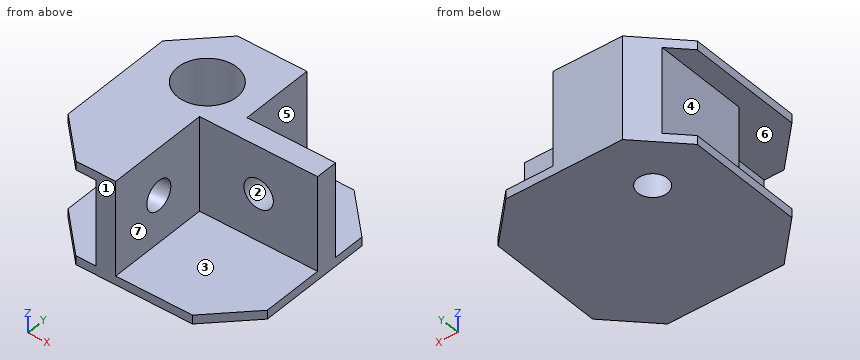
from build123d import *

# Parameters (mm, degrees)
F0_W      = 42.8625
F0_H      = 42.8625
F1_DEPTH  = 22.225
F2_SIZE   = 8.89
F3_W      = 25.4
F3_H      = 22.225
F4_DEPTH  = 20.32
F5_W      = 19.05
F5_H      = 15.875
F6_DEPTH  = 20.32
F8_D      = 12.7
F8_DEPTH  = 20.32
F8_TIP    = 3.8154649308
F9_W      = 14.1852621388
F9_H      = 18.415
F10_DEPTH = 17.78
F11_W     = 6.263975054
F11_H     = 18.415
F12_DEPTH = 25.0835
F14_D     = 6.35
F16_D     = 6.35


with BuildPart() as f1:
    # F0 (on Top) → F1 (new body)
    with BuildSketch(Plane.XY):
        Rectangle(F0_W, F0_H)
    extrude(amount=F1_DEPTH)

    # F2
    f2_edges = [f1.edges().sort_by_distance(p)[0] for p in [
        (-21.43125, -21.43125, 11.1125),
        (21.43125, -21.43125, 11.1125),
        (21.43125, 21.43125, 11.1125),
        (-21.43125, 21.43125, 11.1125),
    ]]
    chamfer(f2_edges, length=F2_SIZE)

    # F3 (on face) → F4 (cut)
    with BuildSketch(Plane.XY.offset(22.225)):
        with Locations((8.73125, -10.31875)):
            Rectangle(F3_W, F3_H)
    extrude(amount=-F4_DEPTH, mode=Mode.SUBTRACT)

    # F5 (on face) → F6 (cut)
    with BuildSketch(Plane.XY.offset(22.225)):
        with Locations((11.90625, 13.49375)):
            Rectangle(F5_W, F5_H)
    extrude(amount=-F6_DEPTH, mode=Mode.SUBTRACT)

    # F8
    with Locations(Plane.XY.offset(22.225)):
        with Locations((-8.73125, 8.73125)):
            Hole(F8_D / 2, depth=F8_DEPTH)
            with Locations((0, 0, -(F8_DEPTH + F8_TIP / 2))):  # 118° drill point
                Cone(0, F8_D / 2, F8_TIP, mode=Mode.SUBTRACT)

    # F9 (on face) → F10 (cut)
    with BuildSketch(Plane.XZ.offset(21.43125)):
        with Locations((-15.3476310694, 11.1125)):
            Rectangle(F9_W, F9_H)
    extrude(amount=-F10_DEPTH, mode=Mode.SUBTRACT)

    # F11 (on face) → F12 (cut, through all)
    with BuildSketch(Plane.XZ.offset(3.65125)):
        with Locations((-20.3739013523, 11.1125)):
            Rectangle(F11_W, F11_H)
    extrude(amount=-F12_DEPTH, mode=Mode.SUBTRACT)

    # F14 (through all)
    with Locations(Plane.YZ.offset(-3.96875)):
        with Locations((-10.00125, 12.065)):
            Hole(F14_D / 2)

    # F16 (through all)
    with Locations(Plane.XZ.offset(-0.79375)):
        with Locations((8.73125, 12.065)):
            Hole(F16_D / 2)


solid = f1.part
Input: part model. Units: mm. Frame: model coordinates. Face numbers are marked on the shaded views. A direction names the side the tool comes from. Coordinates: 2 decimals unless noted, no trailing zeros. Order: outer loops, then holes, each group sorted by start corner. A loop starts at its lowest first (then second) coordinate and runs counter-clockwise, first axis right, second up.
1. Cut plane B-B, the plane y = -0.5. Return loops of the section in (x, z) (3 decimals).
Checked values:
outline: (-21.431, 0) - (21.431, 0) - (21.431, 1.905) - (-3.969, 1.905) - (-3.969, 22.225) - (-21.431, 22.225) - (-21.431, 20.32) - (-17.242, 20.32) - (-17.242, 1.905) - (-21.431, 1.905) - close
2. Cut plane A-A, the plane z = 10. Return loops of the section in (x, y) (3 decimals), plus the area to 3 significant figures.
Checked values:
outline: (-17.242, -3.651) - (-8.255, -3.651) - (-8.255, -7.59) - (-3.969, -7.59) - (-3.969, 0.794) - (6.32, 0.794) - (6.32, 5.556) - (2.381, 5.556) - (2.381, 21.431) - (-12.541, 21.431) - (-17.242, 16.731) - close; (-8.255, -21.431) - (-3.969, -21.431) - (-3.969, -12.413) - (-8.255, -12.413) - close; (11.143, 0.794) - (21.431, 0.794) - (21.431, 5.556) - (11.143, 5.556) - close; hole circle Ø12.7 at (-8.731, 8.731)
area: 450 mm2
3. Cut plane D-D, the plane z = 16.5. Return loops of the section in (x, y) (3 decimals).
Checked values:
outline: (-17.242, -3.651) - (-8.255, -3.651) - (-8.255, -21.431) - (-3.969, -21.431) - (-3.969, 0.794) - (21.431, 0.794) - (21.431, 5.556) - (2.381, 5.556) - (2.381, 21.431) - (-12.541, 21.431) - (-17.242, 16.731) - close; hole circle Ø12.7 at (-8.731, 8.731)
4. Cut plane C-C, the plane x = -16. Return loops of the section in (y, z) (1 decimal), plus the area to 3 significant figures.
Checked values:
outline: (-18, 0) - (18, 0) - (18, 22.2) - (-18, 22.2) - (-18, 20.3) - (-3.7, 20.3) - (-3.7, 1.9) - (-18, 1.9) - close
area: 535 mm2
5. Ray query, line 1 along Z through (x, y) = (-17.5, 2) (3 decimals); line 2 along Y through (x, z) = (13, 14); line 3 along Z through (x, y) = (14, -9.5) (3 decimals). Return the intervals inside material, ascending.
Checked values:
line 1: z = 0 to 1.905, 20.32 to 22.225
line 2: y = 0.79 to 5.56
line 3: z = 0 to 1.905
6. Draft query along Z for the marked faces 1, 2, 3 and 4. Return one class per face: +Z half, -Z half, draft (parallel to the pull), parting line (faces both ways), or undercut.
Checked values:
face 1: draft
face 2: undercut
face 3: +Z half
face 4: undercut
7. Access query for the marked faces 5, 6 and 7. Directions: +Z, -Z, +X, -X, +Y, -Y. A direction counts if a zero-diameter tool reaches every point of the face in a straight line with its end or side. Return the directions, or none.
Checked values:
face 5: +Z, +X, +Y
face 6: -X, -Y
face 7: +Z, +X, -Y
8. Contact query for flat-ended pins moving along their axis: P1, Ø5, axis at y = -10, z = 12.06, coming from the -X side; P2, Ø11, axis at x = 4, y = -11, coming from the +Z side (3 decimals); P3, Ø5.5, axis at y = 10.5, z = 8, coming from the -X side; P4, Ø8, axis at y = 17.5, z = 15, coming from the +X side. Output: stop coordinate, or through.
Checked values:
P1: passes through
P2: stops at z = 1.905
P3: stops at x = -17.24
P4: stops at x = 2.38
